Here's how the part is built. I have some questions about the finished solid (model axes, mm). A direction names the side the tool comes from. Give positions to 0.01 mm unless a question says otherwise; leave off trailing zeros. Order: outer loops, then holes, each group sorted by start corner. A loop starts at its lowest first (then second) coordinate and runs counter-clockwise, first axis right, second up. Notation, with made-up numbers: M 42,22.5 L 71,22.5 A14 cw 71,27.5 Z; hole C 17,85.25 d7. An arc over 180 degrees is marked long. Use CSV: the item, a comma, the result in double quotes. Start each with the question number.
```python
from build123d import *

# Parameters (mm, degrees)
SKETCH1_W                   = 152.4
SKETCH1_H                   = 31.75
BOSS_EXTRUDE1_DEPTH         = 12.7
SKETCH2_W                   = 152.4
SKETCH2_H                   = 11.7475
CUT_EXTRUDE1_DEPTH          = 6.985
F_1_4_20_TAPPED_HOLE1_D     = 5.1054
F_1_4_20_TAPPED_HOLE1_DEPTH = 12.7


with BuildPart() as part:
    # Sketch1 → Boss-Extrude1 (new body)
    with BuildSketch(Plane.XY):
        Rectangle(SKETCH1_W, SKETCH1_H)
    extrude(amount=BOSS_EXTRUDE1_DEPTH)

    # Sketch2 → Cut-Extrude1 (cut)
    with BuildSketch(Plane.XY.offset(12.7)):
        with Locations((0, 10.00125)):
            Rectangle(SKETCH2_W, SKETCH2_H)
        with Locations((0, -10.00125)):
            Rectangle(SKETCH2_W, SKETCH2_H)
    extrude(amount=-CUT_EXTRUDE1_DEPTH, mode=Mode.SUBTRACT)

    # 1/4-20 Tapped Hole1
    with Locations(Plane.XY.offset(12.7)):
        with Locations((-57.15, 0), (-19.05, 0), (19.05, 0), (57.15, 0)):
            Hole(F_1_4_20_TAPPED_HOLE1_D / 2, depth=F_1_4_20_TAPPED_HOLE1_DEPTH)


solid = part.part
```
Q1. Imagine slicing it at A-A, the plane y = 0. Please give me the cut outline in (x, z), then the cut area to 3 significant figures.
Q2. Imagine slicing it at B-B, the plane x = 57.15. Please give me the cut outline in (y, z) (1 decimal), then the cut area to 3 significant figures.
Q3. We'd pull the mould along X, two halves only. Please class faces 4 (the face through (-1, 0, 0)), 5 (the face through (76.2, 0, 5)), 6 (the face through (-54.6, 0.1, 6.3)): pulls with the +X half, pulls with the -X half, needs draft (parallel to the pull), parting line crosses it, or undercut.
Q4. Imagine slicing it at D-D, the plane y = 9. Please give me the cut outline in (x, z) (3 decimals), then the cut area to 3 significant figures.
Q5. For faces 1 (the face through (-1, 4.128, 9)), 2 (the face through (-1, -4.128, 9)), 3 (the face through (-1, -15.875, 3)), which set-ups out of +Z, -Z, +X, -X, +Y, -Y let a thin tool reach every point of the face, with its end or its side?
Q6. I need wall thicknesses on line 1 (Y direction, x = -19.05, z = 5) (3 decimals); line 2 (Y direction, x = 57.15, z = 6); line 3 (Y direction, x = 40.5, z = 10.25). Which ranges of each line are inside material? Lowest first, please. Write a range as [from, to].
Q7. Imagine slicing it at C-C, the plane x = -18. Please give me the cut outline in (y, z) (1 decimal).
Q8. For P1, Ø6.5, axis at x = 19.05, y = 0, coming from the +Z side; P2, Ø7.5, axis at x = -21, z = 10, coming from the +Y side; P3, Ø7.5, axis at x = -0.5, z = 11, coming from the -Y side; P4, Ø9.5, axis at x = -17, y = 11.5, coming from the +Z side (3 decimals), each with a flat end and sliding along its axis, tell me the tip position at first contact or that it passes through.
Reply:
1,outline,"M -76.2,0 L -59.7,0 L -59.7,12.7 L -76.2,12.7 Z; M -54.6,0 L -21.6,0 L -21.6,12.7 L -54.6,12.7 Z; M -16.5,0 L 16.5,0 L 16.5,12.7 L -16.5,12.7 Z; M 21.6,0 L 54.6,0 L 54.6,12.7 L 21.6,12.7 Z; M 59.7,0 L 76.2,0 L 76.2,12.7 L 59.7,12.7 Z"
1,area,"1,680 mm^2"
2,outline,"M -15.9,0 L -2.6,0 L -2.6,12.7 L -4.1,12.7 L -4.1,5.7 L -15.9,5.7 Z; M 2.6,0 L 15.9,0 L 15.9,5.7 L 4.1,5.7 L 4.1,12.7 L 2.6,12.7 Z"
2,area,"174 mm^2"
3,face 4,"needs draft"
3,face 5,"pulls with the +X half"
3,face 6,"undercut"
4,outline,"M -76.2,0 L 76.2,0 L 76.2,5.715 L -76.2,5.715 Z"
4,area,"871 mm^2"
5,face 1,"+Z, +X, -X, +Y"
5,face 2,"+Z, +X, -X, -Y"
5,face 3,"+Z, -Z, +X, -X, -Y"
6,line 1,"y = [-15.875, -2.553], [2.553, 15.875]"
6,line 2,"y = [-4.13, -2.55], [2.55, 4.13]"
6,line 3,"y = [-4.13, 4.13]"
7,outline,"M -15.9,0 L -2.3,0 L -2.3,12.7 L -4.1,12.7 L -4.1,5.7 L -15.9,5.7 Z; M 2.3,0 L 15.9,0 L 15.9,5.7 L 4.1,5.7 L 4.1,12.7 L 2.3,12.7 Z"
8,P1,"stops at z = 12.7"
8,P2,"stops at y = 4.13"
8,P3,"stops at y = -4.13"
8,P4,"stops at z = 5.715"
